Check sheet for the modelled part. Datum: model origin and axes. Units: mm. Coordinates: 2 decimals unless noted, no trailing zeros. Write each loop counter-clockwise with the first axis right and the second up, starting at its lowest first coordinate (ties: lowest second). Pieces come first, ordered by that corner, then holes. Notation, with made-up numbers: (48.5, 21) -> (96.5, 21) arc R15 cw to (96.5, 33) -> close; hole circle Ø6 at (-35, -29). An arc over 180 degrees is marked (long way). One line per item, written item: value. Start each with the question number.
1) Sectioned sample at B-B on z = 1.3. Give the number of separate pieces and of enclosed holes in the cut face, plus the area to 3 significant figures.
2) Gauge pin test, flat ends, axial feed: P1, Ø1.2, axis at x = 80.44, y = 96.73, coming from the -Z side; P2, Ø1.6, axis at x = 252, z = 1, coming from the +Y side. Record the tip position at first contact, or that the pin passes through.
3) Scan lines: line 1 along Y through (x, z) = (340, 2.1); line 2 along X through (y, z) = (205, 2.4); line 3 along X through (y, z) = (144.8, 2.35). Record each from-to range of solid material in increasing order. Write a range as [from, to].
4) Sectioned sample at A-A on x = 314.5. Enter the section's corners in (y, z) (3 decimals), plus the area to 3 significant figures.
```python
from build123d import *

# Parameters (mm, degrees)
F0_R     = 1.025
F0_R_2   = 1.6
F0_W     = 54
F0_H     = 23.811965
F0_W_2   = 8
F0_H_2   = 15
F0_W_3   = 25
F0_H_3   = 8
F0_R_3   = 1.2
F0_R_4   = 2.125
F1_DEPTH = 3.175
F2_R     = 5
F3_R     = 1.25
F4_DEPTH = 3.176


with BuildPart() as f1:
    # F0 (on Top) → F1 (new body)
    with BuildSketch(Plane.XY):
        Polygon((0, 210), (0, 0), (345, 0), (345, 210), (261.513983, 210), (261.513983, 188), (245.513983, 188), (245.513983, 210), align=None)
        with Locations((80.437288, 38.733408)):
            Circle(F0_R, mode=Mode.SUBTRACT)
        with Locations((129.437288, 38.733408)):
            Circle(F0_R, mode=Mode.SUBTRACT)
        with Locations((80.437288, 96.733408)):
            Circle(F0_R, mode=Mode.SUBTRACT)
        with Locations((129.437288, 96.733408)):
            Circle(F0_R, mode=Mode.SUBTRACT)
        with Locations((241.513983, 39.155032)):
            Circle(F0_R_2, mode=Mode.SUBTRACT)
        with Locations((273.513983, 38.532448)):
            Rectangle(F0_W, F0_H, mode=Mode.SUBTRACT)
        with Locations((305.513983, 39.155032)):
            Circle(F0_R_2, mode=Mode.SUBTRACT)
        with Locations((226.013983, 70.155032)):
            Circle(F0_R, mode=Mode.SUBTRACT)
        with Locations((254.013983, 98.155032)):
            Rectangle(F0_W_2, F0_H_2, mode=Mode.SUBTRACT)
        with Locations((306.513983, 68.60377)):
            Rectangle(F0_W_3, F0_H_3, mode=Mode.SUBTRACT)
        with Locations((321.013983, 70.155032)):
            Circle(F0_R, mode=Mode.SUBTRACT)
        with Locations((29.495293, 143.198627)):
            Circle(F0_R_3, mode=Mode.SUBTRACT)
        with Locations((79.495293, 143.198627)):
            Circle(F0_R_3, mode=Mode.SUBTRACT)
        with Locations((129.495293, 143.198627)):
            Circle(F0_R_3, mode=Mode.SUBTRACT)
        with Locations((29.495293, 180.198627)):
            Circle(F0_R_3, mode=Mode.SUBTRACT)
        with Locations((79.495293, 180.198627)):
            Circle(F0_R_3, mode=Mode.SUBTRACT)
        with Locations((129.495293, 180.198627)):
            Circle(F0_R_3, mode=Mode.SUBTRACT)
        with Locations((226.013983, 119.155032)):
            Circle(F0_R, mode=Mode.SUBTRACT)
        with Locations((179.495293, 143.198627)):
            Circle(F0_R_3, mode=Mode.SUBTRACT)
        with Locations((253.513983, 144.8)):
            Circle(F0_R_4, mode=Mode.SUBTRACT)
        with Locations((321.013983, 119.155032)):
            Circle(F0_R, mode=Mode.SUBTRACT)
        with Locations((179.495293, 180.198627)):
            Circle(F0_R_3, mode=Mode.SUBTRACT)
        with Locations((232.513983, 198.5)):
            Circle(F0_R_4, mode=Mode.SUBTRACT)
        with Locations((274.513983, 198.5)):
            Circle(F0_R_4, mode=Mode.SUBTRACT)
    extrude(amount=F1_DEPTH)

    # F2
    f2_edges = [f1.edges().sort_by_distance(p)[0] for p in [
        (0, 210, 1.5875),
        (0, 0, 1.5875),
        (345, 0, 1.5875),
        (345, 210, 1.5875),
    ]]
    fillet(f2_edges, radius=F2_R)

    # F3 (on face) → F4 (cut, through all)
    with BuildSketch(Plane.XY.offset(3.175)):
        with Locations((5, 5)):
            Circle(F3_R)
        with Locations((5, 205)):
            Circle(F3_R)
        with Locations((340, 5)):
            Circle(F3_R)
        with Locations((340, 205)):
            Circle(F3_R)
        with Locations((172.5, 5)):
            Circle(F3_R)
        with Locations((172.5, 205)):
            Circle(F3_R)
    extrude(amount=-F4_DEPTH, mode=Mode.SUBTRACT)


solid = f1.part
```
Answers:
1. separate pieces: 1
1. enclosed holes: 30
1. area: 70,300 mm2
2. P1: passes through
2. P2: stops at y = 188
3. line 1: y = [0, 3.75], [6.25, 203.75], [206.25, 210]
3. line 2: x = [0, 3.75], [6.25, 171.25], [173.75, 245.51], [261.51, 338.75], [341.25, 345]
3. line 3: x = [0, 251.39], [255.64, 345]
4. outline: (0, 0) -> (64.604, 0) -> (64.604, 3.175) -> (0, 3.175) -> close; (72.604, 0) -> (210, 0) -> (210, 3.175) -> (72.604, 3.175) -> close
4. area: 641 mm2
